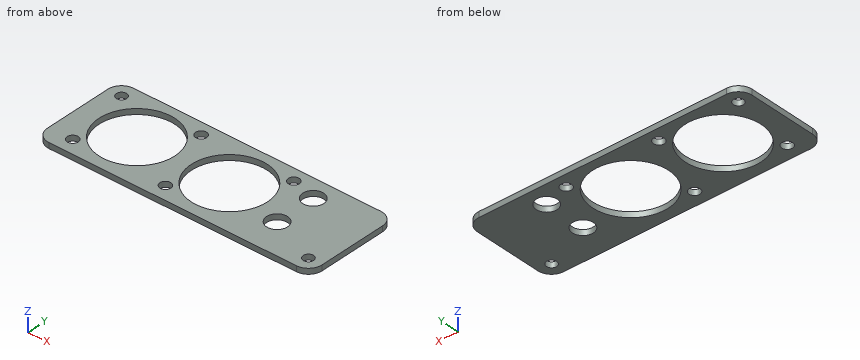
```python
from build123d import *

# Parameters (mm, degrees)
SKETCH1_R           = 11.05
SKETCH1_R_2         = 1.6
SKETCH1_R_3         = 1.5
SKETCH1_R_4         = 3.05
BOSS_EXTRUDE1_DEPTH = 1.6


with BuildPart() as part:
    # Sketch1 → Boss-Extrude1 (new body)
    with BuildSketch(Plane.XY):
        with BuildLine():
            Line((-36, -14), (36, -14))
            ThreePointArc((36, -14), (38.828427125, -12.828427125), (40, -10))
            Line((40, -10), (40, 10))
            ThreePointArc((40, 10), (38.828427125, 12.828427125), (36, 14))
            Line((36, 14), (-36, 14))
            ThreePointArc((-36, 14), (-38.828427125, 12.828427125), (-40, 10))
            Line((-40, 10), (-40, -10))
            ThreePointArc((-40, -10), (-38.828427125, -12.828427125), (-36, -14))
        make_face()
        with Locations((-23, 0.3)):
            Circle(SKETCH1_R, mode=Mode.SUBTRACT)
        with Locations((3.92, 0.3)):
            Circle(SKETCH1_R, mode=Mode.SUBTRACT)
        with Locations((14, 10.2)):
            Circle(SKETCH1_R_2, mode=Mode.SUBTRACT)
        with Locations((-6, -9.6)):
            Circle(SKETCH1_R_2, mode=Mode.SUBTRACT)
        with Locations((-33, -9.6)):
            Circle(SKETCH1_R_2, mode=Mode.SUBTRACT)
        with Locations((-13, 10.2)):
            Circle(SKETCH1_R_2, mode=Mode.SUBTRACT)
        with Locations((-36, 10)):
            Circle(SKETCH1_R_3, mode=Mode.SUBTRACT)
        with Locations((21.6, 8)):
            Circle(SKETCH1_R_4, mode=Mode.SUBTRACT)
        with Locations((21.6, -4)):
            Circle(SKETCH1_R_4, mode=Mode.SUBTRACT)
        with Locations((36, -10)):
            Circle(SKETCH1_R_3, mode=Mode.SUBTRACT)
    extrude(amount=BOSS_EXTRUDE1_DEPTH)


solid = part.part
```
Read the model definition and answer for the solid it produces. Units are mm, in the model's axes. Round coordinates to 2 decimals unless told otherwise and drop trailing zeros. Write each loop counter-clockwise with the first axis right and the second up, starting at its lowest first coordinate (ties: lowest second). Pieces come first, ordered by that corner, then holes. Notation, with made-up numbers: (31, -35.5) -> (83, -35.5) arc R11 cw to (83, -23.5) -> close; hole circle Ø8 at (1.5, 67.25). An arc over 180 degrees is marked (long way). Answer in a Markdown table with one row per item. Add a question column.
1) Find section C-C, the plane y = -2.5. Determine the outline of the cut face in (x, z), and give its area (3 significant figures).
2) Find section B-B, the plane x = -23. Determine the outline of the cut face in (y, z), and give its area (3 significant figures).
3) Consider line 1 (Y direction, x = 21.6, z = 0.85); line 2 (X direction, y = -2.5, z = 0.9); line 3 (Y direction, x = -23, z = 1.1). Determine where each line is inside the solid, lowest interval first.
4) Find section D-D, the plane y = -5.5. Determine the outline of the cut face in (x, z), and give its area (3 significant figures).
5) Find section A-A, the plane z = 0.9. State how many separate pieces and enclosed holes the cut face has, and give its area (3 significant figures).
Findings below:
| question | item | result |
|---|---|---|
| 1 | outline | (-40, 0) -> (-33.69, 0) -> (-33.69, 1.6) -> (-40, 1.6) -> close; (-12.31, 0) -> (-6.77, 0) -> (-6.77, 1.6) -> (-12.31, 1.6) -> close; (14.61, 0) -> (18.94, 0) -> (18.94, 1.6) -> (14.61, 1.6) -> close; (24.26, 0) -> (40, 0) -> (40, 1.6) -> (24.26, 1.6) -> close |
| 1 | area | 51.1 mm² |
| 2 | outline | (-14, 0) -> (-10.75, 0) -> (-10.75, 1.6) -> (-14, 1.6) -> close; (11.35, 0) -> (14, 0) -> (14, 1.6) -> (11.35, 1.6) -> close |
| 2 | area | 9.44 mm² |
| 3 | line 1 | -14 to -7.05, -0.95 to 4.95, 11.05 to 14 |
| 3 | line 2 | -40 to -33.69, -12.31 to -6.77, 14.61 to 18.94, 24.26 to 40 |
| 3 | line 3 | -14 to -10.75, 11.35 to 14 |
| 4 | outline | (-40, 0) -> (-32.41, 0) -> (-32.41, 1.6) -> (-40, 1.6) -> close; (-13.59, 0) -> (-5.49, 0) -> (-5.49, 1.6) -> (-13.59, 1.6) -> close; (13.33, 0) -> (18.94, 0) -> (18.94, 1.6) -> (13.33, 1.6) -> close; (24.26, 0) -> (40, 0) -> (40, 1.6) -> (24.26, 1.6) -> close |
| 4 | area | 59.3 mm² |
| 5 | separate pieces | 1 |
| 5 | enclosed holes | 10 |
| 5 | area | 1,350 mm² |
